from build123d import *

# Parameters (mm, degrees)
F0_W          = 88.9
F0_H          = 88.9
F1_DEPTH      = 88.9
F2_W          = 63.5
F2_H          = 63.5
F3_DEPTH      = 88.9
F4_W          = 88.9
F4_H          = 12.7
F5_DEPTH      = 101.6
F6_R          = 12.7
F7_DEPTH      = 38.1
F8_W          = 7.62
F8_H          = 34.29
F8_H_2        = 7.62
F8_W_2        = 34.29
F9_DEPTH      = 7.62
F10_W         = 76.2
F10_H         = 12.7
F11_DEPTH     = 12.7
F12_W         = 76.2
F12_H         = 12.7
F13_DEPTH     = 12.7
F14_R         = 3.81
F15_DEPTH     = 19.05
F16_W         = 50.8
F16_H         = 12.7
F17_DEPTH     = 25.4
F18_R         = 8.89
F19_T1_DEPTH  = 76.2
F19_T3_DEPTH  = 50.8
F19_T8_DEPTH  = 76.2
F19_S9_R      = 3.81
F19_T10_DEPTH = 40
F19_S11_R     = 3.81
F19_T12_DEPTH = 40
F20_R         = 3.81


# Not quite as in the source:
# - a fillet or chamfer that OpenCascade refuses, or shapes differently, is made with other operations: its cross-section is extruded or revolved along the edge and cut away or added


with BuildPart() as f1:
    # F0 (on Top) → F1 (new body)
    with BuildSketch(Plane.XY):
        Rectangle(F0_W, F0_H)
    extrude(amount=F1_DEPTH)

    # F2 (on face) → F3 (cut)
    with BuildSketch(Plane.YZ.offset(44.45)):
        with Locations((0, 44.45)):
            Rectangle(F2_W, F2_H)
    extrude(amount=-F3_DEPTH, mode=Mode.SUBTRACT)

    # F4 (on face) → F5 (join)
    with BuildSketch(Plane.XY.offset(88.9)):
        with Locations((0, 38.1)):
            Rectangle(F4_W, F4_H)
    extrude(amount=F5_DEPTH)

    # F6 (on face) → F7 (join)
    with BuildSketch(Plane(origin=(0, 0, 0), x_dir=(1, 0, 0), z_dir=(0, 0, -1))):
        Circle(F6_R)
    extrude(amount=F7_DEPTH)

    # F8 (on face) → F9 (join)
    with BuildSketch(Plane(origin=(0, 0, -38.1), x_dir=(1, 0, 0), z_dir=(0, 0, -1))):
        with Locations((0, 20.955)):
            Rectangle(F8_W, F8_H)
        Rectangle(F8_W, F8_H_2)
        with Locations((-20.955, 0)):
            Rectangle(F8_W_2, F8_H_2)
        with Locations((20.955, 0)):
            Rectangle(F8_W_2, F8_H_2)
        with Locations((0, -20.955)):
            Rectangle(F8_W, F8_H)
    extrude(amount=F9_DEPTH)

    # F10 (on face) → F11 (join)
    with BuildSketch(Plane.YZ.offset(44.45)):
        with Locations((6.35, 120.65)):
            Rectangle(F10_W, F10_H)
    extrude(amount=F11_DEPTH)

    # F12 (on face) → F13 (join)
    with BuildSketch(Plane(origin=(-44.45, 0, 0), x_dir=(0, -1, 0), z_dir=(-1, 0, 0))):
        with Locations((-6.35, 120.65)):
            Rectangle(F12_W, F12_H)
    extrude(amount=F13_DEPTH)

    # F14 (on face) → F15 (join)
    with BuildSketch(Plane.XY.offset(190.5)):
        with Locations((19.05, 38.1)):
            Circle(F14_R)
        with Locations((-19.05, 38.1)):
            Circle(F14_R)
    extrude(amount=F15_DEPTH)

    # F16 (on face) → F17 (join)
    with BuildSketch(Plane.XY.offset(209.55)):
        with Locations((0, 38.1)):
            Rectangle(F16_W, F16_H)
    extrude(amount=F17_DEPTH)

    # F18
    f18_edges = [f1.edges().sort_by_distance(p)[0] for p in [
        (0, -44.45, 88.9),
    ]]
    fillet(f18_edges, radius=F18_R)

    # F19: fillet of radius 5.08 on 4 edges, made by hand

    # F19_s2 → F19_t1 (cut)
    with BuildSketch(Plane.YZ.offset(-38.1)):
        with BuildLine():
            ThreePointArc((31.75, 229.87), (33.2378975516, 233.4621024484), (36.83, 234.95))
            Line((36.83, 234.95), (31.75, 234.95))
            Line((31.75, 234.95), (31.75, 229.87))
        make_face()
    extrude(amount=F19_T1_DEPTH, mode=Mode.SUBTRACT)

    # F19_s4 → F19_t3 (cut)
    with BuildSketch(Plane.XY.offset(196.85)):
        with BuildLine():
            ThreePointArc((20.32, 31.75), (23.9121024484, 33.2378975516), (25.4, 36.83))
            Line((25.4, 36.83), (25.4, 31.75))
            Line((25.4, 31.75), (20.32, 31.75))
        make_face()
        with BuildLine():
            ThreePointArc((-20.32, 31.75), (-23.9121024484, 33.2378975516), (-25.4, 36.83))
            Line((-25.4, 36.83), (-25.4, 31.75))
            Line((-25.4, 31.75), (-20.32, 31.75))
        make_face()
    extrude(amount=F19_T3_DEPTH, mode=Mode.SUBTRACT)


with BuildPart() as f19_tool6:
    # F19_s7 → F19_t8 (new body)
    with BuildSketch(Plane.YZ.offset(-38.1)):
        with BuildLine():
            ThreePointArc((36.83, 209.55), (33.2378975516, 211.0378975516), (31.75, 214.63))
            Line((31.75, 214.63), (31.75, 209.55))
            Line((31.75, 209.55), (36.83, 209.55))
        make_face()
    extrude(amount=F19_T8_DEPTH)

    # F19_s9 → F19_t10 (cut, symmetric)
    with BuildSketch(Plane.XY.offset(212.1)):
        with Locations((-19.05, 38.1)):
            Circle(F19_S9_R)
    extrude(amount=F19_T10_DEPTH, both=True, mode=Mode.SUBTRACT)

    # F19_s11 → F19_t12 (cut, symmetric)
    with BuildSketch(Plane.XY.offset(212.1)):
        with Locations((19.05, 38.1)):
            Circle(F19_S11_R)
    extrude(amount=F19_T12_DEPTH, both=True, mode=Mode.SUBTRACT)


with BuildPart() as f1_1:
    add(f1.part)

    # F19_t5: cut F19_tool6
    add(f19_tool6.part, mode=Mode.SUBTRACT)

    # F20
    f20_edges = [f1_1.edges().sort_by_distance(p)[0] for p in [
        (44.45, 0, 127),
        (57.15, 6.35, 127),
        (-44.45, 0, 127),
        (-57.15, 6.35, 127),
    ]]
    fillet(f20_edges, radius=F20_R)


solid = f1_1.part
Verification items for the finished model (mm, model axes). A direction names the side the tool comes from. Give positions to 0.01 mm unless a question says otherwise; leave off trailing zeros. Loops run counter-clockwise (first coordinate to the right, second up) from the corner with the lowest first, then second, coordinate; pieces in that order, holes last.
1. Cross-section at D-D on x = 0. Record the cut outline in (y, z).
Derived:
outline: (-44.45, 0) - (-12.7, 0) - (-12.7, -38.1) - (-38.1, -38.1) - (-38.1, -45.72) - (38.1, -45.72) - (38.1, -38.1) - (12.7, -38.1) - (12.7, 0) - (44.45, 0) - (44.45, 190.5) - (31.75, 190.5) - (31.75, 88.9) - (-35.56, 88.9) arc R8.89 ccw to (-44.45, 80.01) - close; (31.75, 214.63) arc R5.08 ccw to (36.83, 209.55) - (44.45, 209.55) - (44.45, 234.95) - (36.83, 234.95) arc R5.08 ccw to (31.75, 229.87) - close; hole (-31.75, 12.7) - (31.75, 12.7) - (31.75, 76.2) - (-31.75, 76.2) - close
2. Go/stop test with flat-tipped pins: P1, Ø4, axis at y = 2, z = -43, coming from the +X side; P2, Ø6.5, axis at x = -48, y = 21.5, coming from the -Z side; P3, Ø4, axis at y = -20.5, z = -40, coming from the -X side. Record where each tip stops, or that it passes through.
Derived:
P1: stops at x = 38.1
P2: stops at z = 114.3
P3: stops at x = -3.81
3. Release check for a two-part mould opening along Y. For faces 4 (the cylindrical face through (23.872, 33.199, 222.072)), 5 (the flat face through (-7, 7, -38.1)), 6 (the flat face through (1, -31.75, 44)) record: +Y half, -Y half, draft (parallel to the pull), parting line (faces both ways), or undercut.
Derived:
face 4: -Y half
face 5: draft
face 6: undercut
4. Cross-section at A-A on x = 28. Record the cut outline in (y, z).
Derived:
outline: (-44.45, 0) - (44.45, 0) - (44.45, 190.5) - (31.75, 190.5) - (31.75, 88.9) - (-35.56, 88.9) arc R8.89 ccw to (-44.45, 80.01) - close; (-3.81, -45.72) - (3.81, -45.72) - (3.81, -38.1) - (-3.81, -38.1) - close; hole (-31.75, 12.7) - (31.75, 12.7) - (31.75, 76.2) - (-31.75, 76.2) - close
5. Cross-section at C-C on y = -19. Record the cut outline in (x, z), and give its area (3 significant figures).
Derived:
outline: (-57.15, 114.3) - (-44.45, 114.3) - (-44.45, 123.19) arc R3.81 ccw to (-48.26, 127) - (-53.34, 127) arc R3.81 ccw to (-57.15, 123.19) - close; (-44.45, 0) - (44.45, 0) - (44.45, 12.7) - (-44.45, 12.7) - close; (-44.45, 76.2) - (44.45, 76.2) - (44.45, 88.9) - (-44.45, 88.9) - close; (-3.81, -45.72) - (3.81, -45.72) - (3.81, -38.1) - (-3.81, -38.1) - close; (44.45, 114.3) - (57.15, 114.3) - (57.15, 123.19) arc R3.81 ccw to (53.34, 127) - (48.26, 127) arc R3.81 ccw to (44.45, 123.19) - close
area: 2,630 mm2
6. Material ranges on probe 1 along Z at (x, y) = (-1, -33); probe 2 along Y at (x, z) = (-11, 57); probe 3 along Z at (x, y) = (-28, -20), recorded low to high.
Derived:
probe 1: z = -45.72 to -38.1, 0 to 88.9
probe 2: y = -44.45 to -31.75, 31.75 to 44.45
probe 3: z = 0 to 12.7, 76.2 to 88.9
7. Tool access check on faces 1 (the flat face through (44.45, 0, 119)), 2 (the flat face through (-3.81, -21, -42)), 3 (the flat face through (51, 6, 127)). Record the directions out of +Z, -Z, +X, -X, +Y, -Y that give a thin tool (end or side, any length) a straight path to the whole face; none if there is none.
Derived:
face 1: +Z, -Y
face 2: -Z, -X, -Y
face 3: +Z, +X, +Y, -Y
8. Cross-section at B-B on y = 0. Record the cut outline in (x, z).
Derived:
outline: (-57.15, 114.3) - (-44.45, 114.3) - (-44.45, 123.19) arc R3.81 ccw to (-48.26, 127) - (-53.34, 127) arc R3.81 ccw to (-57.15, 123.19) - close; (-44.45, 0) - (-12.7, 0) - (-12.7, -38.1) - (-38.1, -38.1) - (-38.1, -45.72) - (38.1, -45.72) - (38.1, -38.1) - (12.7, -38.1) - (12.7, 0) - (44.45, 0) - (44.45, 12.7) - (-44.45, 12.7) - close; (-44.45, 76.2) - (44.45, 76.2) - (44.45, 88.9) - (-44.45, 88.9) - close; (44.45, 114.3) - (57.15, 114.3) - (57.15, 123.19) arc R3.81 ccw to (53.34, 127) - (48.26, 127) arc R3.81 ccw to (44.45, 123.19) - close
